from build123d import *

# Parameters (mm, degrees)
SKETCH_1_R               = 19
EXTRUDE_1_DEPTH          = 30
SKETCH_2_R               = 8
EXTRUDE_2_DEPTH          = 22
SKETCH_3_R               = 10
CUT_EXTRUDE_1_DEPTH      = 67.670833355
CUT_EXTRUDE_2_REACH      = 56.24
CUT_EXTRUDE_2_END_RADIUS = 10
SKETCH_4_R               = 4
EXTRUDE_START            = -74
SKETCH_5_W               = 90
SKETCH_5_H               = 80
EXTRUDE_3_DEPTH          = 12
FILLET_1_R               = 10
SKETCH_6_W               = 30
SKETCH_6_H               = 80
CUT_EXTRUDE_3_DEPTH      = 4
CUT_EXTRUDE_4_DEPTH      = 164.740648637
EXTRUDE_4_DEPTH          = 4
EXTRUDE_5_DEPTH          = 20
FILLET_2_R               = 10


with BuildPart() as part:
    # Sketch 1 → Extrude 1 (new, symmetric)
    with BuildSketch(Plane.XY):
        Circle(SKETCH_1_R)
    extrude(amount=EXTRUDE_1_DEPTH, both=True)

    # Sketch 2 → Extrude 2 (add)
    with BuildSketch(Plane(origin=(0, 0, 0), x_dir=(1, 0, 0), z_dir=(0, 1, 0))):
        with Locations(Location((0, 0, 0), (0, 0, 90))):
            Circle(SKETCH_2_R)
    extrude(amount=EXTRUDE_2_DEPTH)

    # Sketch 3 → Cut-Extrude 1 (cut, through all)
    with BuildSketch(Plane.XY.offset(30)):
        Circle(SKETCH_3_R)
    extrude(amount=-CUT_EXTRUDE_1_DEPTH, mode=Mode.SUBTRACT)

    # Cut-Extrude 2: up to this cylinder (the profile starts outside it)
    cut_extrude_2_end = Plane(origin=(0, 0, 0), z_dir=(0, 0, 1)) * Cylinder(CUT_EXTRUDE_2_END_RADIUS, 133.48, mode=Mode.PRIVATE)
    # Sketch 4 → Cut-Extrude 2 (cut, up to the surface)
    with BuildSketch(Plane(origin=(0, 22, 0), x_dir=(1, 0, 0), z_dir=(0, 1, 0)), mode=Mode.PRIVATE) as cut_extrude_2_sk1:
        with Locations(Location((0, 0, 0), (0, 0, 270))):
            Circle(SKETCH_4_R)
    cut_extrude_2_tool1 = extrude(cut_extrude_2_sk1.sketch, amount=-CUT_EXTRUDE_2_REACH, mode=Mode.PRIVATE) - cut_extrude_2_end
    add(cut_extrude_2_tool1.solids().sort_by_distance((0, 22, 0))[0], mode=Mode.SUBTRACT)



with BuildPart() as body_2:
    # Sketch 5 → Extrude 3 (new body)
    with BuildSketch(Plane(origin=(0, 0, 0), x_dir=(0, 0, -1), z_dir=(1, 0, 0)).offset(EXTRUDE_START)):
        with Locations((0, -95)):
            Rectangle(SKETCH_5_W, SKETCH_5_H)
    extrude(amount=EXTRUDE_3_DEPTH)

    # Fillet 1
    fillet_1_edges = [body_2.edges().sort_by_distance(p)[0] for p in [
        (-68, -135, -45),
        (-68, -135, 45),
        (-68, -55, 45),
        (-68, -55, -45),
    ]]
    fillet(fillet_1_edges, radius=FILLET_1_R)

    # Sketch 6 → Cut-Extrude 3 (cut)
    with BuildSketch(Plane.ZY.offset(74)):
        with Locations((0, -95)):
            Rectangle(SKETCH_6_W, SKETCH_6_H)
    extrude(amount=-CUT_EXTRUDE_3_DEPTH, mode=Mode.SUBTRACT)

    # Sketch 7 → Cut-Extrude 4 (cut, through all)
    with BuildSketch(Plane(origin=(-62, 0, 0), x_dir=(0, 0, -1), z_dir=(1, 0, 0))):
        with BuildLine():
            Line((-26, -85), (-26, -105))
            ThreePointArc((-26, -105), (-30, -109), (-34, -105))
            Line((-34, -105), (-34, -85))
            ThreePointArc((-34, -85), (-30, -81), (-26, -85))
        make_face()
    cut_extrude_4 = extrude(amount=-CUT_EXTRUDE_4_DEPTH, mode=Mode.SUBTRACT)

    # Mirror 1: Cut-Extrude 4 across plane
    add(cut_extrude_4.mirror(Plane.XY), mode=Mode.SUBTRACT)


with BuildPart() as part_1:
    add(part.part)

    add(body_2.part)  # Extrude 4 merges body 2
    # Sketch 8 → Extrude 4 (add, symmetric)
    with BuildSketch(Plane.XY):
        with BuildLine():
            Line((-19, 0), (-19, -25))
            ThreePointArc((-19, -25), (-27.786796564, -46.213203436), (-49, -55))
            Line((-49, -55), (-62, -55))
            Line((-62, -55), (-62, -117))
            ThreePointArc((-62, -117), (-57.554804791, -102.769750529), (-45.8, -93.6))
            ThreePointArc((-45.8, -93.6), (1.219219164, -56.920997883), (19, 0))
            ThreePointArc((19, 0), (0, -19), (-19, 0))
        make_face()
    extrude(amount=EXTRUDE_4_DEPTH, both=True)

    # Sketch 9 → Extrude 5 (add, symmetric)
    with BuildSketch(Plane.XY):
        with BuildLine():
            Line((-49, -55), (-62, -55))
            Line((-62, -55), (-62, -73))
            ThreePointArc((-62, -73), (-59.071067812, -65.928932188), (-52, -63))
            Line((-52, -63), (-49, -63))
            ThreePointArc((-49, -63), (-22.129942315, -51.870057685), (-11, -25))
            Line((-11, -25), (-11, -15.491933385))
            ThreePointArc((-11, -15.491933385), (-16.881943016, -8.717797887), (-19, 0))
            Line((-19, 0), (-19, -25))
            ThreePointArc((-19, -25), (-27.786796564, -46.213203436), (-49, -55))
        make_face()
    extrude(amount=EXTRUDE_5_DEPTH, both=True)

    # Fillet 2
    # the kernel refuses this fillet: 10 mm, written as the material it adds along each edge
    with BuildSketch(Plane(origin=(-11, -15.491933385, -20), x_dir=(0.9464272027660603, -0.32291724925189497, 0), z_dir=(0, 0, 1))) as fillet_2_piece_1_section:
        with BuildLine():
            CenterArc((13.662534862, -9.586356274), FILLET_2_R, 106.537100336, 87.550188329)
            Line((3.963274477, -12.020354626), (2.993348438, -12.263754461))
            ThreePointArc((2.993348438, -12.263754461), (2.123891514, -9.32161014), (-0.946427203, -0.322917249))
            Line((-0.946427203, -0.322917249), (0.284636143, 0.958635627))
            ThreePointArc((0.284636143, 0.958635627), (5.408086716, 0.214076921), (10.531537289, 0.958635627))
            Line((10.531537289, 0.958635627), (10.816173432, 0))
        make_face()
    fillet_2_piece_1 = extrude(amount=47.642186032, mode=Mode.PRIVATE)
    fillet_2_piece_1 = split(fillet_2_piece_1, bisect_by=Plane(origin=(-8.746000777, -19.792422089, 20), z_dir=(0, 0, -1)), keep=Keep.TOP, mode=Mode.PRIVATE)
    add(fillet_2_piece_1)
    with BuildSketch(Plane(origin=(-11, -15.491933385, -27.642186032), x_dir=(0.9464272027660603, -0.32291724925189513, 0), z_dir=(0, 0, 1))) as fillet_2_piece_2_section:
        with BuildLine():
            CenterArc((13.662534862, -9.586356274), FILLET_2_R, 106.537100336, 87.550188329)
            Line((3.963274477, -12.020354626), (2.993348438, -12.263754461))
            ThreePointArc((2.993348438, -12.263754461), (2.123891514, -9.32161014), (-0.946427203, -0.322917249))
            Line((-0.946427203, -0.322917249), (0.284636143, 0.958635627))
            ThreePointArc((0.284636143, 0.958635627), (5.408086716, 0.214076921), (10.531537289, 0.958635627))
            Line((10.531537289, 0.958635627), (10.816173432, 0))
        make_face()
    fillet_2_piece_2 = extrude(amount=47.642186032, mode=Mode.PRIVATE)
    fillet_2_piece_2 = split(fillet_2_piece_2, bisect_by=Plane(origin=(-8.746000777, -19.792422089, -20), z_dir=(0, 0, 1)), keep=Keep.TOP, mode=Mode.PRIVATE)
    add(fillet_2_piece_2)


solid = part_1.part
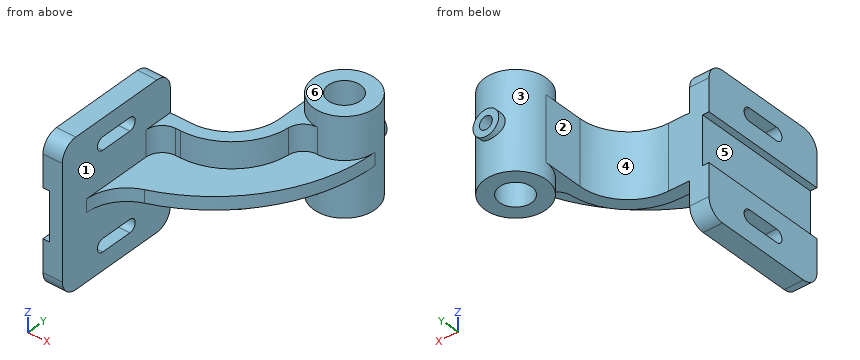
Build history of the part. All positions in model axes, mm. Face numbers are marked on the shaded views. A direction names the side the tool comes from. Give positions to 0.01 mm unless a question says otherwise; leave off trailing zeros. Order: outer loops, then holes, each group sorted by start corner. A loop starts at its lowest first (then second) coordinate and runs counter-clockwise, first axis right, second up. Notation, with made-up numbers: M 15,18.25 L 19,18.25 A16 cw 19,32.25 Z; hole C 10,11 d7. An arc over 180 degrees is marked long. Use one line per item in the form item = value.
Q1. Wall check: probe 1 along Y at (x, z) = (0, -15); probe 2 along X at (y, z) = (-87, -20); probe 3 along Z at (x, y) = (0, -51.5). Give the ranges that are in metal, low to high.
Conclusion:
probe_1 = -19 to -10, 10 to 19
probe_2 = -74 to -62
probe_3 = -4 to 4
Q2. Which spindle directions (+Z, -Z, +X, -X, +Y, -Y) get a long thin tool onto all of the face, cutting with end or side? Do the marked faces 1, 2 and 3. Say none if no direction does.
Conclusion:
face_1 = +X, -Y
face_2 = +Z, -Z, -X, +Y
face_3 = none
Q3. Slice it at A-A, the plane z = 28. Write the cut outline in (x, y), and give its area (3 significant figures).
Conclusion:
outline = M -74,-135 L -62,-135 L -62,-108.46 L -74,-108.46 Z; M -74,-81.54 L -62,-81.54 L -62,-55 L -74,-55 Z; C 0,0 d38; hole C 0,0 d20
area = 1,460 mm2
Q4. Slice it at D-D, the plane y = 6. Write the cut outline in (x, z).
Conclusion:
outline = M -18.03,-30 L -8,-30 L -8,30 L -18.03,30 Z; M 8,-30 L 18.03,-30 L 18.03,30 L 8,30 Z
Q5. Pull direction Z, two halves, no side cores. Call the marked faces 4, 5 and 6: released by +Z, released by -Z, zero draft, split by the parting line, or undercut.
Conclusion:
face_4 = zero draft
face_5 = undercut
face_6 = released by +Z
Q6. Pin check, flat tips, straight feed: P1, Ø24, axis at y = -94.5, z = 2.5, coming from the +X side; P2, Ø0.9, axis at x = -50, z = -8.5, coming from the -Y side; P3, Ø19, axis at x = 4, y = 9.5, coming from the +Z side; P4, Ø10, axis at x = -40, y = -46, coming from the +Z side. Stop position of each tip, or through.
Conclusion:
P1 = -24.49
P2 = -63
P3 = 30
P4 = through
Q7. Slice it at B-B, the plane y = -103. Write the cut outline in (x, z).
Conclusion:
outline = M -74,-45 L -62,-45 L -62,-34 L -74,-34 Z; M -74,-26 L -62,-26 L -62,-4 L -57.71,-4 L -57.71,4 L -62,4 L -62,26 L -74,26 L -74,15 L -70,15 L -70,-15 L -74,-15 Z; M -74,34 L -62,34 L -62,45 L -74,45 Z
Q8. Slice it at C-C, the plane z = 0. Write the cut outline in (x, y).
Conclusion:
outline = M -70,-135 L -62,-135 L -62,-117 A25 cw -45.8,-93.6 A100 ccw 19,0 A19 ccw 8,17.23 L 8,22 L 4,22 L 4,9.17 A10 cw long -4,9.17 L -4,22 L -8,22 L -8,17.23 A19 ccw -19,0 L -19,-25 A30 cw -49,-55 L -70,-55 Z
